```python
from build123d import *

# Parameters (mm, degrees)
CROQUIS1_W              = 65
CROQUIS1_H              = 65
CROQUIS1_W_2            = 49
CROQUIS1_H_2            = 49
SALIENTE_EXTRUIR1_DEPTH = 28
CROQUIS2_R              = 11.115
CORTAR_EXTRUIR1_DEPTH   = 5
CROQUIS3_R              = 5.155
CORTAR_EXTRUIR2_DEPTH   = 8
CROQUIS5_R              = 6.5
CORTAR_EXTRUIR3_DEPTH   = 5
CROQUIS6_R              = 3
CORTAR_EXTRUIR4_DEPTH   = 5
CROQUIS7_R              = 3.175
CORTAR_EXTRUIR5_DEPTH   = 5


with BuildPart() as part:
    # Croquis1 → Saliente-Extruir1 (new body)
    with BuildSketch(Plane.XY):
        with Locations((32.5, 32.5)):
            Rectangle(CROQUIS1_W, CROQUIS1_H)
        with Locations((32.5, 32.5)):
            Rectangle(CROQUIS1_W_2, CROQUIS1_H_2, mode=Mode.SUBTRACT)
    extrude(amount=SALIENTE_EXTRUIR1_DEPTH)

    # Croquis2 → Cortar-Extruir1 (cut)
    with BuildSketch(Plane.ZY):
        with Locations((14, 32.5)):
            Circle(CROQUIS2_R)
    extrude(amount=-CORTAR_EXTRUIR1_DEPTH, mode=Mode.SUBTRACT)

    # Croquis3 → Cortar-Extruir2 (cut)
    with BuildSketch(Plane.ZY):
        with Locations((14, 32.5)):
            Circle(CROQUIS3_R)
    extrude(amount=-CORTAR_EXTRUIR2_DEPTH, mode=Mode.SUBTRACT)

    # Croquis5 → Cortar-Extruir3 (cut)
    with BuildSketch(Plane.ZY.offset(-57)):
        with Locations((14, 32.5)):
            Circle(CROQUIS5_R)
    extrude(amount=-CORTAR_EXTRUIR3_DEPTH, mode=Mode.SUBTRACT)

    # Croquis6 → Cortar-Extruir4 (cut)
    with BuildSketch(Plane(origin=(0, 65, 0), x_dir=(1, 0, 0), z_dir=(0, 1, 0))):
        with Locations(Location((32.5, -14, 0), (0, 0, 270))):
            Circle(CROQUIS6_R)
    extrude(amount=-CORTAR_EXTRUIR4_DEPTH, mode=Mode.SUBTRACT)

    # Croquis7 → Cortar-Extruir5 (cut)
    with BuildSketch(Plane.XZ):
        with Locations(Location((32.5, 14, 0), (0, 0, 270))):
            Circle(CROQUIS7_R)
    extrude(amount=-CORTAR_EXTRUIR5_DEPTH, mode=Mode.SUBTRACT)


solid = part.part
```
Part model, mm, in its own coordinate system. A direction names the side the tool comes from. Round coordinates to 2 decimals unless told otherwise and drop trailing zeros. Write each loop counter-clockwise with the first axis right and the second up, starting at its lowest first coordinate (ties: lowest second). Pieces come first, ordered by that corner, then holes.
Item 1: Cut at C-C, the plane z = 14. Give the cut face in (x, y) (3 decimals).
Results:
outline: (0, 0) - (29.325, 0) - (29.325, 5) - (35.675, 5) - (35.675, 0) - (65, 0) - (65, 65) - (35.5, 65) - (35.5, 60) - (29.5, 60) - (29.5, 65) - (0, 65) - (0, 43.615) - (5, 43.615) - (5, 37.655) - (8, 37.655) - (8, 57) - (57, 57) - (57, 39) - (62, 39) - (62, 26) - (57, 26) - (57, 8) - (8, 8) - (8, 27.345) - (5, 27.345) - (5, 21.385) - (0, 21.385) - close
Item 2: Cut at A-A, the plane x = 17.5. Give the cut face in (y, z).
Results:
outline: (0, 0) - (8, 0) - (8, 28) - (0, 28) - close; (57, 0) - (65, 0) - (65, 28) - (57, 28) - close
Item 3: Which spindle directions (+Z, -Z, +X, -X, +Y, -Y) get a long thin tool onto all of the face, cutting with end or side? Do faces 4 (the cylindrical face through (29.7, 2.5, 12.5)), 5 (the cylindrical face through (59.465, 38.945, 13.154)), 6 (the flat face through (33, 60, 14)). Say none if no direction does.
Results:
face 4: -Y
face 5: none
face 6: +Y
Item 4: Cut at D-D, the plane x = 6. Give the cut face in (y, z) (3 decimals), plus the area to 3 significant figures.
Results:
outline: (0, 0) - (65, 0) - (65, 28) - (0, 28) - close; hole circle Ø10.31 at (32.5, 14)
area: 1,740 mm2
Item 5: Two-plate mould, pull along Z, no slides. Class faces 1 (the cylindrical face through (34.53, 62.54, 11.79)), 2 (the flat face through (3, 33, 0)), 3 (the flat face through (32, 8, 14)): +Z half, -Z half, draft (parallel to the pull), parting line (faces both ways), or undercut.
Results:
face 1: undercut
face 2: -Z half
face 3: draft
Item 6: Cut at B-B, the plane y = 32.5. Give the cut face in (x, z) (3 decimals), plus the area to 3 significant figures.
Results:
outline: (0, 0) - (8, 0) - (8, 8.845) - (5, 8.845) - (5, 2.885) - (0, 2.885) - close; (0, 25.115) - (5, 25.115) - (5, 19.155) - (8, 19.155) - (8, 28) - (0, 28) - close; (57, 0) - (65, 0) - (65, 28) - (57, 28) - (57, 20.5) - (62, 20.5) - (62, 7.5) - (57, 7.5) - close
area: 241 mm2
Item 7: Probe L1, parallel to Y at x = 21, z = 13.5; L2, parallel to X at y = 23.5, z = 12.5; L3, parallel to Z at x = 60, y = 32. List the from-to ranges inside material, lowest first.
Results:
L1: y = 0 to 8, 57 to 65
L2: x = 5 to 8, 57 to 65
L3: z = 0 to 7.52, 20.48 to 28
Item 8: Drop flat-ended pins along their axis: pin 1 Ø3 at (x, z) = (32.5, 13) entering from +Y; pin 2 Ø4 at (x, z) = (13, 25) entering from -Y; pin 3 Ø11 at (y, z) = (33, 10) entering from -X; pin 4 Ø5 at (x, z) = (32.5, 14) entering from -Y. Give the stop position or say it passes through.
Results:
pin 1: stops at y = 60
pin 2: stops at y = 0
pin 3: stops at x = 5
pin 4: stops at y = 5
